Part print with two shaded views. Sizes in mm from the minimum x, y, z corner. A direction names the side the tool comes from. Round coordinates to 2 decimals unless told otherwise and drop trailing zeros. Loops run counter-clockwise (first coordinate to the right, second up) from the corner with the lowest first, then second, coordinate; pieces in that order, holes last.
(1) Mould opens along X. For the marked faces 1, 2, 3 and 4 say: +X half, -X half, draft (parallel to the pull), parting line (faces both ways), or undercut.
(2) Probe probe 1 along Y at (x, z) = (8.89, 3.5); probe 2 along X at (y, z) = (5, 12) (1 decimal); probe 3 along Z at (x, y) = (10.5, 7). List the from-to ranges inside material, lowest first.
(3) Tool access for the marked faces 5 and 6: list every direction of +Z, -Z, +X, -X, +Y, -Y with a clear straight run to the whole face (end or side of a thin tool).
(4) Cut at D-D on z = 30. List the corners of the cut face in (x, y).
(5) Cut at A-A on z = 8. Count the separate pieces of the cut face and the enclosed holes in it, then the cut area to 3 significant figures.
(6) Flat gauge pins, fed straight in: pin 1 (2.5 mm diameter, centred on x = 8.89, y = 5.08, fed in from +Z); pin 2 (5 mm diameter, centred on x = 78.74, y = 77.47, fed in from -Z); pin 3 (1.9 mm diameter, centred on x = 9.5, y = 3.5, fed in from +Z); pin 4 (3 mm diameter, centred on y = 68.5, z = 32, fed in from +X). Where does each tip first touch, or does it go through?
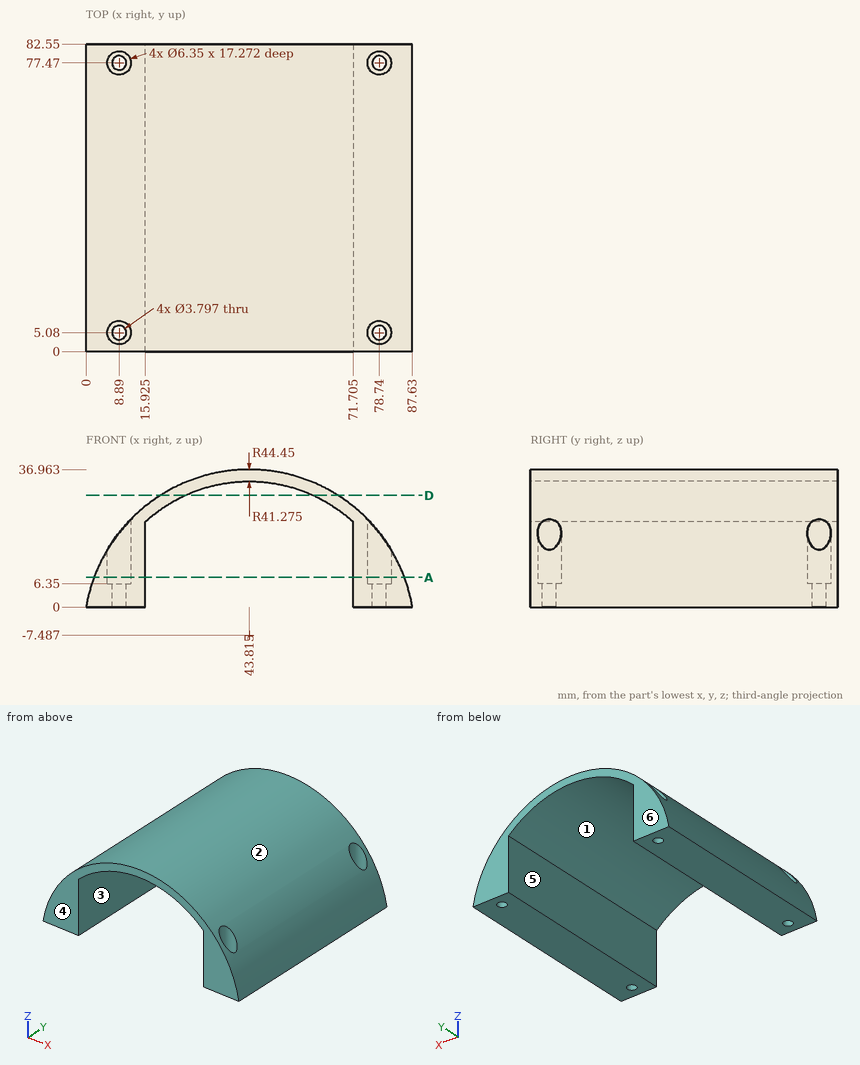
Final values:
1. face 1: undercut
1. face 2: parting line
1. face 3: undercut
1. face 4: draft
2. probe 1: y = 0 to 3.18, 6.98 to 75.57, 79.37 to 82.55
2. probe 2: x = 3.9 to 5.7, 12.1 to 15.9, 71.7 to 75.6, 81.9 to 83.8
2. probe 3: z = 0 to 6.35
3. face 5: -Z, +Y, -Y
3. face 6: +Z, -Z, +X, -X, +Y
4. outline: (19.93, 0) - (26.54, 0) - (26.54, 82.55) - (19.93, 82.55) - close; (61.09, 0) - (67.7, 0) - (67.7, 82.55) - (61.09, 82.55) - close
5. separate pieces: 2
5. enclosed holes: 4
5. area: 2,150 mm2
6. pin 1: passes through
6. pin 2: stops at z = 0
6. pin 3: stops at z = 6.35
6. pin 4: stops at x = 66.9
